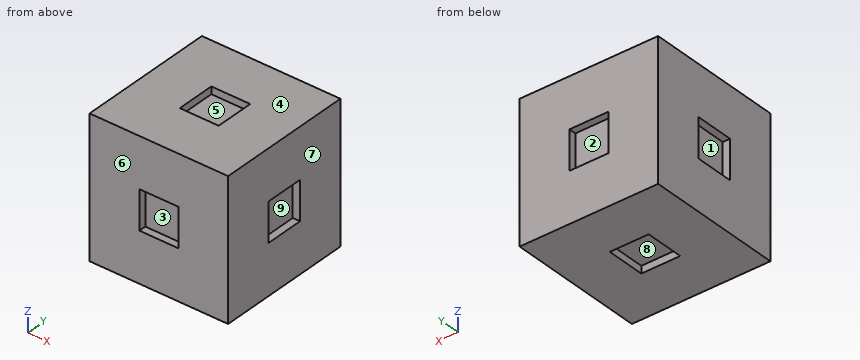
```python
from build123d import *

# Parameters (mm, degrees)
SKETCH_1_W          = 57
SKETCH_1_H          = 57
EXTRUDE_1_DEPTH     = 57
SKETCH_2_W          = 16
SKETCH_2_H          = 16
CUT_EXTRUDE_1_DEPTH = 3
SKETCH_3_W          = 16
SKETCH_3_H          = 16
CUT_EXTRUDE_2_DEPTH = 3
SKETCH_4_W          = 16
SKETCH_4_H          = 16
CUT_EXTRUDE_3_DEPTH = 3
SKETCH_5_W          = 16
SKETCH_5_H          = 16
CUT_EXTRUDE_4_DEPTH = 3
SKETCH_6_W          = 16
SKETCH_6_H          = 16
CUT_EXTRUDE_5_DEPTH = 3
SKETCH_7_W          = 16
SKETCH_7_H          = 16
CUT_EXTRUDE_6_DEPTH = 3


with BuildPart() as part:
    # 草图1 → 凸台-拉伸1 (new body)
    with BuildSketch(Plane(origin=(0, 0, 0), x_dir=(1, 0, 0), z_dir=(0, 1, 0))):
        Rectangle(SKETCH_1_W, SKETCH_1_H)
    extrude(amount=EXTRUDE_1_DEPTH)

    # 草图2 → 切除-拉伸1 (cut)
    with BuildSketch(Plane.XY.offset(28.5)):
        with Locations((0, 28.5)):
            Rectangle(SKETCH_2_W, SKETCH_2_H)
    extrude(amount=-CUT_EXTRUDE_1_DEPTH, mode=Mode.SUBTRACT)

    # 草图3 → 切除-拉伸2 (cut)
    with BuildSketch(Plane(origin=(28.5, 0, 0), x_dir=(0, 0, -1), z_dir=(1, 0, 0))):
        with Locations((0, 28.5)):
            Rectangle(SKETCH_3_W, SKETCH_3_H)
    extrude(amount=-CUT_EXTRUDE_2_DEPTH, mode=Mode.SUBTRACT)

    # 草图4 → 切除-拉伸3 (cut)
    with BuildSketch(Plane(origin=(0, 0, -28.5), x_dir=(-1, 0, 0), z_dir=(0, 0, -1))):
        with Locations((0, 28.5)):
            Rectangle(SKETCH_4_W, SKETCH_4_H)
    extrude(amount=-CUT_EXTRUDE_3_DEPTH, mode=Mode.SUBTRACT)

    # 草图5 → 切除-拉伸4 (cut)
    with BuildSketch(Plane.ZY.offset(28.5)):
        with Locations((0, 28.5)):
            Rectangle(SKETCH_5_W, SKETCH_5_H)
    extrude(amount=-CUT_EXTRUDE_4_DEPTH, mode=Mode.SUBTRACT)

    # 草图6 → 切除-拉伸5 (cut)
    with BuildSketch(Plane(origin=(0, 57, 0), x_dir=(1, 0, 0), z_dir=(0, 1, 0))):
        Rectangle(SKETCH_6_W, SKETCH_6_H)
    extrude(amount=-CUT_EXTRUDE_5_DEPTH, mode=Mode.SUBTRACT)

    # 草图7 → 切除-拉伸6 (cut)
    with BuildSketch(Plane.XZ):
        Rectangle(SKETCH_7_W, SKETCH_7_H)
    extrude(amount=-CUT_EXTRUDE_6_DEPTH, mode=Mode.SUBTRACT)


solid = part.part
```
Geometry check sheet. Reference: the model listing, model coordinates, mm. Face numbers are marked on the shaded views. A direction names the side the tool comes from. Coordinates: 2 decimals unless noted, no trailing zeros. Order: outer loops, then holes, each group sorted by start corner. A loop starts at its lowest first (then second) coordinate and runs counter-clockwise, first axis right, second up. Notation, with made-up numbers: (6.5, 14.5) - (12.5, 14.5) arc R17 cw to (12.5, 44.5) - close; hole circle Ø5 at (-7.75, 34.25). An arc over 180 degrees is marked (long way). Answer in a Markdown table with one row per item. Add a question column.
1. Section check A-A (z = -4.5). Enter the section's corners in (x, y).
2. Draft check along Y on the marked faces 1, 2, 3 and 4. Enter one of: +Y half, -Y half, draft (parallel to the pull), parting line (faces both ways), or undercut.
3. Gauge pin test, flat end, axial feed: pin 1 Ø8 at (x, z) = (3.5, 2.5) entering from -Y. Record the tip position at first contact, or that the pin passes through.
4. Material ranges on L1, parallel to Z at x = 4, y = 26.5; L2, parallel to Y at x = 5, z = 2, recorded low to high. Write a range as [from, to].
5. Section check B-B (y = 25.5). Enter the section's corners in (x, z), plus the area to 3 significant figures.
6. Access from +Z, -Z, +X, -X, +Y, -Y to the whole of each face (thin tool, end or side, straight path). Record for the marked faces 5, 6, 7, 8 and 9.
Data:
| question | item | result |
|---|---|---|
| 1 | outline | (-28.5, 0) - (-8, 0) - (-8, 3) - (8, 3) - (8, 0) - (28.5, 0) - (28.5, 20.5) - (25.5, 20.5) - (25.5, 36.5) - (28.5, 36.5) - (28.5, 57) - (8, 57) - (8, 54) - (-8, 54) - (-8, 57) - (-28.5, 57) - (-28.5, 36.5) - (-25.5, 36.5) - (-25.5, 20.5) - (-28.5, 20.5) - close |
| 2 | face 1 | undercut |
| 2 | face 2 | +Y half |
| 2 | face 3 | -Y half |
| 2 | face 4 | draft |
| 3 | pin 1 | stops at y = 3 |
| 4 | L1 | z = [-25.5, 25.5] |
| 4 | L2 | y = [3, 54] |
| 5 | outline | (-28.5, -28.5) - (-8, -28.5) - (-8, -25.5) - (8, -25.5) - (8, -28.5) - (28.5, -28.5) - (28.5, -8) - (25.5, -8) - (25.5, 8) - (28.5, 8) - (28.5, 28.5) - (8, 28.5) - (8, 25.5) - (-8, 25.5) - (-8, 28.5) - (-28.5, 28.5) - (-28.5, 8) - (-25.5, 8) - (-25.5, -8) - (-28.5, -8) - close |
| 5 | area | 3,060 mm² |
| 6 | face 5 | +Z |
| 6 | face 6 | +Z, -Z, +X, -X, -Y |
| 6 | face 7 | +Z, -Z, +X, +Y, -Y |
| 6 | face 8 | -Z |
| 6 | face 9 | +X |
